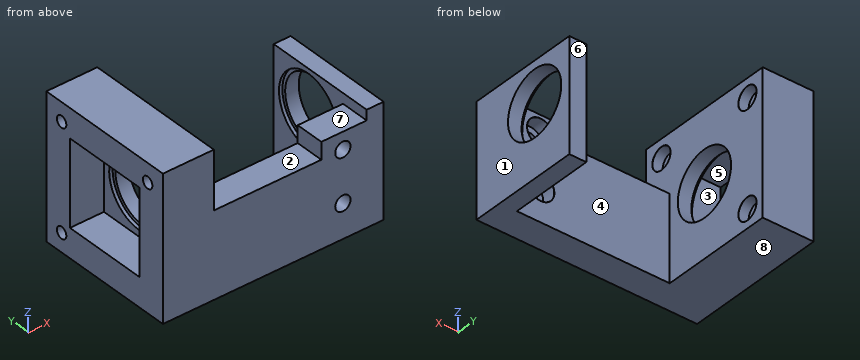
from build123d import *

# Parameters (mm, degrees)
SKETCH1_W                     = 55
SKETCH1_H                     = 33
BOSS_EXTRUDE1_DEPTH           = 5
SKETCH2_W                     = 5
SKETCH2_H                     = 24
BOSS_EXTRUDE2_DEPTH           = 25
HOLE1_D                       = 19.2
HOLE1_DEPTH                   = 5
HOLE1_CBORE_D                 = 21.2
HOLE1_CBORE_DEPTH             = 1
HOLE2_D                       = 19.2
HOLE2_DEPTH                   = 5
HOLE2_CBORE_D                 = 21.2
HOLE2_CBORE_DEPTH             = 1
BOSS_EXTRUDE3_DEPTH           = 5
SKETCH13_W                    = 42
SKETCH13_H                    = 42
SKETCH13_W_2                  = 25
SKETCH13_H_2                  = 25
BOSS_EXTRUDE4_DEPTH           = 10
CBORE_FOR_M3_SHCS3_AT_2_COUNT = 2
CBORE_FOR_M3_SHCS3_AT_2_PITCH = 31
CBORE_FOR_M3_SHCS3_AT_3_COUNT = 2
CBORE_FOR_M3_SHCS3_AT_3_PITCH = 43.840620434
SKETCH23_W                    = 50
SKETCH23_H                    = 33
BOSS_EXTRUDE6_DEPTH           = 3.5
CBORE_FOR_M4_SHCS1_AT_2_COUNT = 2
CBORE_FOR_M4_SHCS1_AT_2_PITCH = 15
CUT_EXTRUDE3_DEPTH            = 57.380404397
SKETCH24_W                    = 5
SKETCH24_H                    = 9
BOSS_EXTRUDE7_DEPTH           = 25


with BuildPart() as part:
    # Sketch1 → Boss-Extrude1 (new body)
    with BuildSketch(Plane(origin=(0, 0, 0), x_dir=(1, 0, 0), z_dir=(0, 1, 0))):
        Rectangle(SKETCH1_W, SKETCH1_H)
    extrude(amount=BOSS_EXTRUDE1_DEPTH)

    # Sketch2 → Boss-Extrude2 (add)
    with BuildSketch(Plane(origin=(0, 5, 0), x_dir=(1, 0, 0), z_dir=(0, 1, 0))):
        with Locations((-25, -4.5)):
            Rectangle(SKETCH2_W, SKETCH2_H)
        with Locations((25, -4.5)):
            Rectangle(SKETCH2_W, SKETCH2_H)
    extrude(amount=BOSS_EXTRUDE2_DEPTH)

    # Hole1
    with Locations(Plane(origin=(-27.5, 0, 0), x_dir=(0, 0, -1), z_dir=(-1, 0, 0))):
        with Locations((-4.5, -17.5)):
            CounterBoreHole(HOLE1_D / 2, HOLE1_CBORE_D / 2, HOLE1_CBORE_DEPTH, depth=HOLE1_DEPTH)

    # Hole2
    with Locations(Plane(origin=(22.5, 0, 0), x_dir=(0, 0, -1), z_dir=(-1, 0, 0))):
        with Locations((-4.5, -17.5)):
            CounterBoreHole(HOLE2_D / 2, HOLE2_CBORE_D / 2, HOLE2_CBORE_DEPTH, depth=HOLE2_DEPTH)

    # Sketch12 → Boss-Extrude3 (add)
    with BuildSketch(Plane.ZY.offset(27.5)):
        Polygon((-16.5, 38.5), (25.5, 38.5), (25.5, -3.5), (-16.5, -3.5), (-16.5, 0), (16.5, 0), (16.5, 30), (-7.5, 30), (-7.5, 5), (-16.5, 5), align=None)
    extrude(amount=-BOSS_EXTRUDE3_DEPTH)

    # Sketch13 → Boss-Extrude4 (add)
    with BuildSketch(Plane.ZY.offset(27.5)):
        with Locations((4.5, 17.5)):
            Rectangle(SKETCH13_W, SKETCH13_H)
        with Locations((4.5, 17.5)):
            Rectangle(SKETCH13_W_2, SKETCH13_H_2, mode=Mode.SUBTRACT)
    extrude(amount=BOSS_EXTRUDE4_DEPTH)

    # Sketch15 → CBORE for M3 SHCS3 (revolve, cut)
    with BuildSketch(Plane(origin=(-22.5, 2, 20), x_dir=(0, 0, -1), z_dir=(0, 1, 0))):
        Polygon((0, 0), (0, 15), (1.7, 15), (1.7, 3), (3.25, 3), (3.25, 0.020977491), (3.275, 0), align=None)
    cbore_for_m3_shcs3 = revolve(axis=Axis((-16.15, 2, 20), (-1, 0, 0)), mode=Mode.SUBTRACT)

    # CBORE for M3 SHCS3 at 2: CBORE for M3 SHCS3 ×2
    with Locations(*[(0, i * CBORE_FOR_M3_SHCS3_AT_2_PITCH, 0) for i in range(1, CBORE_FOR_M3_SHCS3_AT_2_COUNT)]):
        add(cbore_for_m3_shcs3, mode=Mode.SUBTRACT)

    # CBORE for M3 SHCS3 at 3: CBORE for M3 SHCS3 ×2
    with Locations(*[Vector(0, 0.7071067811865476, -0.7071067811865476) * (i * CBORE_FOR_M3_SHCS3_AT_3_PITCH) for i in range(1, CBORE_FOR_M3_SHCS3_AT_3_COUNT)]):
        add(cbore_for_m3_shcs3, mode=Mode.SUBTRACT)

    # Sketch23 → Boss-Extrude6 (add)
    with BuildSketch(Plane.XZ):
        with Locations((2.5, 0)):
            Rectangle(SKETCH23_W, SKETCH23_H)
    extrude(amount=BOSS_EXTRUDE6_DEPTH)

    # Sketch10 → CBORE for M4 SHCS1 (revolve, cut)
    with BuildSketch(Plane(origin=(15.5, 5, -6.5), x_dir=(0, 0, 1), z_dir=(1, 0, 0))):
        Polygon((0, 0), (0, 8.5), (2.25, 8.5), (2.25, 4), (4, 4), (4, 0.020977491), (4.025, 0), align=None)
    cbore_for_m4_shcs1 = revolve(axis=Axis((15.5, 11.35, -6.5), (0, -1, 0)), mode=Mode.SUBTRACT)

    # CBORE for M4 SHCS1 at 2: CBORE for M4 SHCS1 ×2
    with Locations(*[(0, 0, i * CBORE_FOR_M4_SHCS1_AT_2_PITCH) for i in range(1, CBORE_FOR_M4_SHCS1_AT_2_COUNT)]):
        add(cbore_for_m4_shcs1, mode=Mode.SUBTRACT)

    # Sketch21 → Cut-Extrude3 (cut, through all)
    with BuildSketch(Plane(origin=(0, 5, 0), x_dir=(1, 0, 0), z_dir=(0, 1, 0))):
        Polygon((-22.5, -16.5), (-22.5, -8.5), (9.15, -8.5), (9.15, -13.5), (22.5, -13.5), (22.5, -16.5), align=None)
    extrude(amount=-CUT_EXTRUDE3_DEPTH, mode=Mode.SUBTRACT)

    # Sketch24 → Boss-Extrude7 (add)
    with BuildSketch(Plane(origin=(0, 5, 0), x_dir=(1, 0, 0), z_dir=(0, 1, 0))):
        with Locations((25, 12)):
            Rectangle(SKETCH24_W, SKETCH24_H)
    extrude(amount=BOSS_EXTRUDE7_DEPTH)


solid = part.part
Geometry check sheet. Reference: the model listing, model coordinates, mm. Face numbers are marked on the shaded views. A direction names the side the tool comes from. Give positions to 0.01 mm unless a question says otherwise; leave off trailing zeros. Order: outer loops, then holes, each group sorted by start corner. A loop starts at its lowest first (then second) coordinate and runs counter-clockwise, first axis right, second up.
1. Sectioned sample at B-B (x = -29). Record the boundary of the cut face in (y, z), then the cut area to 3 significant figures.
Completed:
outline: (-3.5, -16.5) - (38.5, -16.5) - (38.5, 25.5) - (-3.5, 25.5) - close; hole circle Ø3.4 at (2, 20); hole (5, -8) - (30, -8) - (30, 17) - (5, 17) - close; hole circle Ø3.4 at (33, -11); hole circle Ø3.4 at (33, 20)
area: 1,110 mm2
2. Sectioned sample at A-A (y = 33). Record the boundary of the cut face in (x, z) (3 decimals).
Completed:
outline: (-37.5, -16.5) - (-22.5, -16.5) - (-22.5, -14.275) - (-22.521, -14.25) - (-25.5, -14.25) - (-25.5, -12.7) - (-37.5, -12.7) - close; (-37.5, -9.3) - (-25.5, -9.3) - (-25.5, -7.75) - (-22.521, -7.75) - (-22.5, -7.725) - (-22.5, 16.725) - (-22.521, 16.75) - (-25.5, 16.75) - (-25.5, 18.3) - (-37.5, 18.3) - close; (-37.5, 21.7) - (-25.5, 21.7) - (-25.5, 23.25) - (-22.521, 23.25) - (-22.5, 23.275) - (-22.5, 25.5) - (-37.5, 25.5) - close
3. Draft check along Z on the marked faces 5, 6, 7 and 8. Enter one of: pulls with the +Z half, pulls with the -Z half, needs draft (parallel to the pull), parting line crosses it, or undercut.
Completed:
face 5: undercut
face 6: needs draft
face 7: pulls with the +Z half
face 8: pulls with the -Z half
4. Scan lines: line 1 (Y direction, x = -31.25, z = 20); line 2 (X direction, y = 15, z = -11.5); line 3 (X direction, y = 8, z = 10.5). Record each from-to range of solid material in increasing order.
Completed:
line 1: y = -3.5 to 0.3, 3.7 to 31.3, 34.7 to 38.5
line 2: x = -37.5 to -22.5, 22.5 to 27.5
line 3: x = -27.5 to -22.5, 22.5 to 27.5
5. Depth check by flat-ended pin: pin 1 (1 mm diameter, centred on x = 2.5, y = 4.5, fed in from +Z); pin 2 (12 mm diameter, centred on x = 17, z = -4.5, fed in from +Y); pin 3 (1.5 mm diameter, centred on x = 15, z = 13.5, fed in from +Y); pin 4 (15.5 mm diameter, centred on y = 17.5, z = 4.5, fed in from -X). Enter the tip coordinate at first touch or a pass-through.
Completed:
pin 1: stops at z = 8.5
pin 2: stops at y = 30
pin 3: stops at y = 5
pin 4: passes through
6. Sectioned sample at C-C (y = 6). Record the boundary of the cut face in (x, z).
Completed:
outline: (-37.5, -16.5) - (-22.5, -16.5) - (-22.5, 25.5) - (-37.5, 25.5) - (-37.5, 17) - (-27.5, 17) - (-27.5, -8) - (-37.5, -8) - close; (22.5, -16.5) - (27.5, -16.5) - (27.5, 16.5) - (22.5, 16.5) - close
7. Access from +Z, -Z, +X, -X, +Y, -Y to the whole of each face (thin tool, end or side, straight path). Record for the marked faces 1, 2, 3 and 4.
Completed:
face 1: +Z, -Z, +X, +Y, -Y
face 2: +Z, +Y, -Y
face 3: -X
face 4: +Z, -Z, +Y
8. Sectioned sample at D-D (z = 20). Record the boundary of the cut face in (x, y) (3 decimals), then the cut area to 3 significant figures.
Completed:
outline: (-37.5, -3.5) - (-22.5, -3.5) - (-22.5, -1.275) - (-22.521, -1.25) - (-25.5, -1.25) - (-25.5, 0.3) - (-37.5, 0.3) - close; (-37.5, 3.7) - (-25.5, 3.7) - (-25.5, 5.25) - (-22.521, 5.25) - (-22.5, 5.275) - (-22.5, 29.725) - (-22.521, 29.75) - (-25.5, 29.75) - (-25.5, 31.3) - (-37.5, 31.3) - close; (-37.5, 34.7) - (-25.5, 34.7) - (-25.5, 36.25) - (-22.521, 36.25) - (-22.5, 36.275) - (-22.5, 38.5) - (-37.5, 38.5) - close
area: 509 mm2
